from build123d import *

# Parameters (mm, degrees)
BOSS_EXTRUDE1_DEPTH     = 25.4
SKETCH3_W               = 16.407631331
SKETCH3_H               = 10.16
BOSS_EXTRUDE2_DEPTH     = 25.4
FILLET1_R               = 5.08
SKETCH4_R               = 2.54
CUT_EXTRUDE1_DEPTH      = 44.18
CUT_EXTRUDE1_DEPTH_BACK = 11.16


with BuildPart() as part:
    # Sketch1 → Boss-Extrude1 (new body)
    with BuildSketch(Plane.XY):
        with BuildLine():
            Line((-53.34, 0), (-46.99, 0))
            ThreePointArc((-46.99, 0), (0, 46.99), (46.99, 0))
            Line((46.99, 0), (53.34, 0))
            ThreePointArc((53.34, 0), (0, 53.34), (-53.34, 0))
        make_face()
    extrude(amount=BOSS_EXTRUDE1_DEPTH)

    # Sketch3 → Boss-Extrude2 (add)
    with BuildSketch(Plane(origin=(0, 0, 0), x_dir=(-1, 0, 0), z_dir=(0, 0, -1))):
        with Locations((55.193815666, 5.08)):
            Rectangle(SKETCH3_W, SKETCH3_H)
        with Locations((-55.398553003, 5.08)):
            Rectangle(SKETCH3_W, SKETCH3_H)
    extrude(amount=-BOSS_EXTRUDE2_DEPTH)

    # Fillet1
    fillet1_edges = [part.edges().sort_by_distance(p)[0] for p in [
        (-52.363441445, 10.16, 12.7),
        (52.363441445, 10.16, 12.7),
    ]]
    fillet(fillet1_edges, radius=FILLET1_R)

    # Sketch4 → Cut-Extrude1 (cut, two sides)
    with BuildSketch(Plane(origin=(0, 10.16, 0), x_dir=(1, 0, 0), z_dir=(0, 1, 0))) as cut_extrude1_sk:
        with Locations((-56.39715241, -12.7)):
            Circle(SKETCH4_R)
        with Locations((56.39715241, -12.7)):
            Circle(SKETCH4_R)
    extrude(amount=CUT_EXTRUDE1_DEPTH, mode=Mode.SUBTRACT)
    extrude(cut_extrude1_sk.sketch, amount=-CUT_EXTRUDE1_DEPTH_BACK, mode=Mode.SUBTRACT)


solid = part.part
Input: part model. Units: mm. Frame: model coordinates. A direction names the side the tool comes from. Round coordinates to 2 decimals unless told otherwise and drop trailing zeros. Write each loop counter-clockwise with the first axis right and the second up, starting at its lowest first coordinate (ties: lowest second). Pieces come first, ordered by that corner, then holes.
1) Ray query, L1, parallel to X at y = 4.5, z = 12.7; L2, parallel to X at y = 6.5, z = 12.7; L3, parallel to Y at x = 1, z = 8.25. Return the intervals inside material, ascending.
2) Draft query along X for faces 4 (the cylindrical face through (-1.03, 46.98, 12.52)), 5 (the flat face through (-10, 47, 0)), 6 (the cylindrical face through (53.272, 11.235, 12.522)). Return one class per face: pulls with the +X half, pulls with the -X half, needs draft (parallel to the pull), parting line crosses it, or undercut.
3) Reachability of faces 1 (the cylindrical face through (0.98, 53.33, 12.52)), 2 (the flat face through (-60, 10.16, 13)), 3 (the flat face through (60, 10.16, 13)) from +Z, -Z, +X, -X, +Y, -Y: full face, straight path, thin tool, end or side. Return the list, or none.
4) Cut plane D-D (y = 16.5). Return the cut outline in (x, z), then the cut area to 3 significant figures.
5) Contact query for flat-ended pins moving along their axis: P1, Ø3, axis at x = 56.4, z = 12.7, coming from the -Y side; P2, Ø3, axis at y = 29.5, z = 5, coming from the +X side; P3, Ø1.5, axis at y = 20, z = 12, coming from the -X side; P4, Ø3, axis at y = 31, z = 19.5, coming from the -X side. Output: stop coordinate, or through.
6) Cut plane B-B (y = 28.5). Return the cut outline in (x, z).
7) Cut plane A-A (z = 12.7). Return the cut outline in (x, y), then the cut area to 3 significant figures.
8) Cut plane C-C (z = 22). Return the cut outline in (x, y).
Geometry says:
1. L1: x = -63.4 to -58.94, -53.86 to -46.77, 46.77 to 53.86, 58.94 to 63.6
1. L2: x = -63.4 to -58.94, -53.86 to -46.54, 46.54 to 53.86, 58.94 to 63.6
1. L3: y = 46.98 to 53.33
2. face 4: undercut
2. face 5: needs draft
2. face 6: pulls with the +X half
3. face 1: +Z, -Z, +Y
3. face 2: +Z, -Z, -X, +Y
3. face 3: +Z, -Z, +X, +Y
4. outline: (-50.72, 0) - (-44, 0) - (-44, 25.4) - (-50.72, 25.4) - close; (44, 0) - (50.72, 0) - (50.72, 25.4) - (44, 25.4) - close
4. area: 342 mm2
5. P1: passes through
5. P2: stops at x = 45.4
5. P3: stops at x = -49.75
5. P4: stops at x = -44.44
6. outline: (-45.09, 0) - (-37.36, 0) - (-37.36, 25.4) - (-45.09, 25.4) - close; (37.36, 0) - (45.09, 0) - (45.09, 25.4) - (37.36, 25.4) - close
7. outline: (-63.4, 0) - (-58.94, 0) - (-58.94, 10.16) - (-63.4, 10.16) - close; (-53.86, 0) - (-46.99, 0) arc R46.99 cw to (46.99, 0) - (53.86, 0) - (53.86, 10.84) arc R5.08 cw to (51.49, 13.91) arc R53.34 ccw to (-51.49, 13.91) arc R5.08 cw to (-53.86, 10.84) - close; (58.94, 0) - (63.6, 0) - (63.6, 10.16) - (58.94, 10.16) - close
7. area: 1,120 mm2
8. outline: (-63.4, 0) - (-46.99, 0) arc R46.99 cw to (46.99, 0) - (63.6, 0) - (63.6, 10.16) - (56.4, 10.16) arc R5.08 cw to (51.49, 13.91) arc R53.34 ccw to (-51.49, 13.91) arc R5.08 cw to (-56.4, 10.16) - (-63.4, 10.16) - close
